Input: dimensioned drawing with shaded views. Units: mm. Origin: part minimum x, y, z. Give positions to 0.01 mm unless a question says otherwise; leave off trailing zeros. Write each loop counter-clockwise with the first axis right and the second up, starting at its lowest first coordinate (ties: lowest second). Pieces come first, ordered by that corner, then holes.
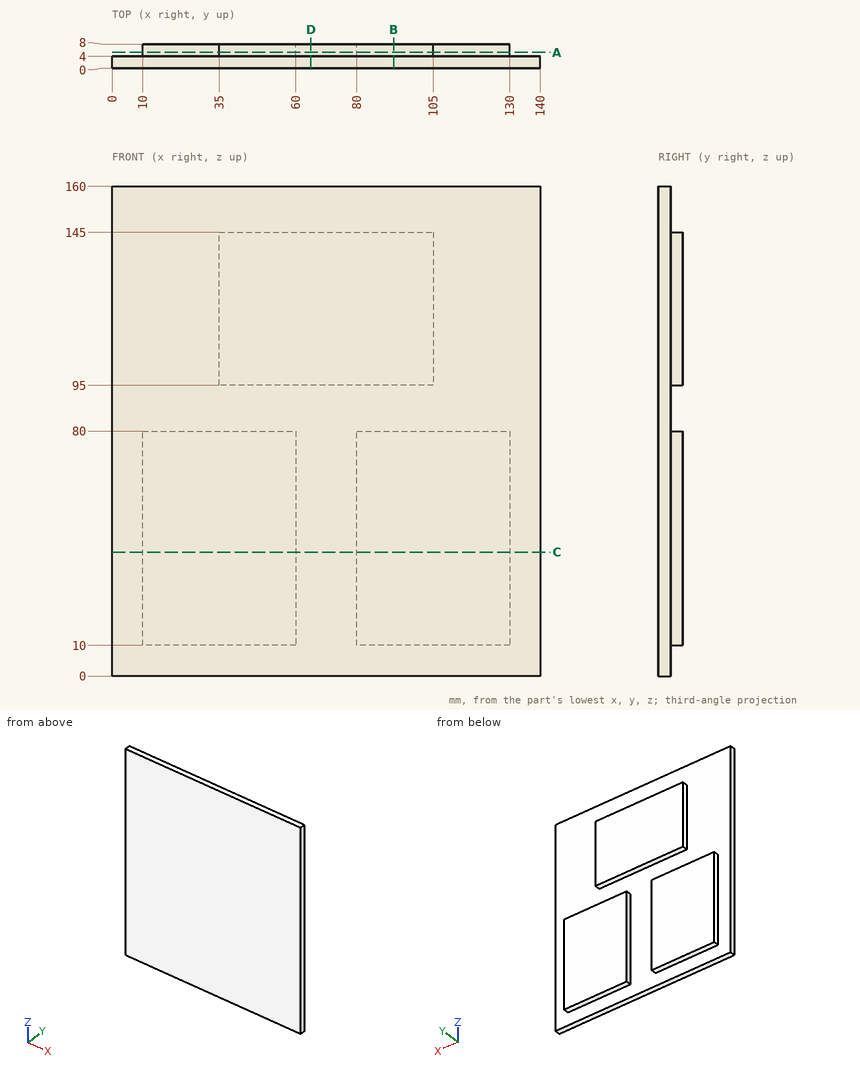
Item 1: Section D-D, the plane x = 65. Return the cut outline in (y, z), plus the area to 3 significant figures.
Found:
outline: (0, 0) - (4, 0) - (4, 95) - (8, 95) - (8, 145) - (4, 145) - (4, 160) - (0, 160) - close
area: 840 mm2
Item 2: Pin query (flat end, axial travel): pin 1 Ø4.5 at (x, y) = (102.5, 6.5) entering from -Z; pin 2 Ø1.2 at (y, z) = (6.5, 47.5) entering from +X; pin 3 Ø4.5 at (y, z) = (7, 54) entering from -X. Return the tip coordinate at first contact, or that it passes through.
Found:
pin 1: stops at z = 10
pin 2: stops at x = 130
pin 3: stops at x = 10
Item 3: Section B-B, the plane x = 92. Return the cut outline in (y, z).
Found:
outline: (0, 0) - (4, 0) - (4, 10) - (8, 10) - (8, 80) - (4, 80) - (4, 95) - (8, 95) - (8, 145) - (4, 145) - (4, 160) - (0, 160) - close
Item 4: Section A-A, the plane y = 5.25. Return the cut outline in (x, z), plus the area to 3 significant figures.
Found:
outline: (10, 10) - (60, 10) - (60, 80) - (10, 80) - close; (35, 95) - (105, 95) - (105, 145) - (35, 145) - close; (80, 10) - (130, 10) - (130, 80) - (80, 80) - close
area: 10,500 mm2
Item 5: Line query: L1, parallel to X at y = 6.25, z = 14; L2, parallel to Y at x = 7.5, z = 16.5; L3, parallel to Z at x = 39, y = 7. Output: solid intervals per line, ascending.
Found:
L1: x = 10 to 60, 80 to 130
L2: y = 0 to 4
L3: z = 10 to 80, 95 to 145
Item 6: Section C-C, the plane z = 40.5. Return the cut outline in (x, y).
Found:
outline: (0, 0) - (140, 0) - (140, 4) - (130, 4) - (130, 8) - (80, 8) - (80, 4) - (60, 4) - (60, 8) - (10, 8) - (10, 4) - (0, 4) - close
